from build123d import *

# Parameters (mm, degrees)
BOSS_EXTRUDE1_DEPTH = 12.446
SKETCH2_R           = 1.450000021
SKETCH2_R_2         = 2.900000042
CUT_EXTRUDE1_DEPTH  = 100.851652202
CHAMFER2_SIZE       = 0.5
CHAMFER3_SIZE       = 1


with BuildPart() as part:
    # Sketch1 → Boss-Extrude1 (new body)
    with BuildSketch(Plane.XY):
        Polygon((0, 8.001), (-41.850200018, 8.001), (-41.850200018, 16.256), (-57.090200018, 16.256), (-82.490200018, 16.256), (-97.730200018, 16.256), (-97.730200018, 8.001), (-97.730200018, -4.699), (-82.490200018, -4.699), (-82.490200018, 8.001), (-54.550200018, 8.001), (-54.550200018, -4.699), (-39.310200018, -4.699), (-39.310200018, 3.302), (-7.874, 3.302), (-7.874, 0), (0, 0), align=None)
    extrude(amount=BOSS_EXTRUDE1_DEPTH)

    # Sketch2 → Cut-Extrude1 (cut, through all)
    with BuildSketch(Plane.XZ):
        with Locations(Location((-90.110200018, 6.223, 0), (0, 0, 270))):
            Circle(SKETCH2_R)
        with Locations(Location((-46.930200018, 6.223, 0), (0, 0, 270))):
            Circle(SKETCH2_R_2)
        with Locations(Location((-3.937, 6.223, 0), (0, 0, 270))):
            Circle(SKETCH2_R)
    extrude(amount=-CUT_EXTRUDE1_DEPTH, mode=Mode.SUBTRACT)

    # Chamfer2
    chamfer2_edges = [part.edges().sort_by_distance(p)[0] for p in [
        (-90.110200018, 16.256, 7.673000021),
        (-3.937, 8.001, 7.673000021),
    ]]
    chamfer(chamfer2_edges, length=CHAMFER2_SIZE)

    # Chamfer3
    chamfer3_edges = [part.edges().sort_by_distance(p)[0] for p in [
        (-46.930200018, 16.256, 9.123000042),
    ]]
    chamfer(chamfer3_edges, length=CHAMFER3_SIZE)


solid = part.part
Work out the finished part from the listing and answer in its coordinate system (mm). A direction names the side the tool comes from. Coordinates: 2 decimals unless noted, no trailing zeros. Order: outer loops, then holes, each group sorted by start corner. A loop starts at its lowest first (then second) coordinate and runs counter-clockwise, first axis right, second up. Notation, with made-up numbers: (8, 3.5) - (51, 3.5) arc R22 cw to (51, 32.5) - close; hole circle Ø2 at (77.5, 87). An arc over 180 degrees is marked (long way). Put each result on its own line as item: value. Start each with the question number.
1) Find section C-C (z = 11). Give the vertices of the cut face in (x, y).
2) Find the intervals of material crossed by line 1 (X direction, y = 7.75, z = 2.25); line 2 (X direction, y = -0.75, z = 0.75); line 3 (X direction, y = 3.75, z = 6), in increasing order. Write a range as from..to.
3) Find section B-B (y = 6). Give the vertices of the cut face in (x, z), plus the area to 3 significant figures.
4) Flat-ended cylindrical pins translate along their axes: pin 1 (3.5 mm diameter, centred on x = -65.5, z = 9, fed in from -Y); pin 2 (0.9 mm diameter, centred on x = -91, z = 7, fed in from +Y); pin 3 (4 mm diameter, centred on x = -5, z = 8, fed in from -Y). Find the tip coordinate at first contact, or state that the pin passes through.
5) For a pull along Z with two mould halves and no side action, classify faces 1 (the flat face through (-60.4, 8.3, 0)), 2 (the flat face through (-90, -4.699, 6)), 3 (the flat face through (-47, 0, 6)) as released by +Z, released by -Z, zero draft, split by the parting line, or undercut.
6) Find section A-A (y = -2.25). Give the vertices of the cut face in (x, z).
7) For faces 4 (the flat face through (-24, 3.302, 6)), 5 (the flat face through (-47, -4.699, 6)), 6 (the flat face through (-21, 8.001, 6)), 7 (the flat face through (-90, 0, 6)), determine the directions among +Z, -Z, +X, -X, +Y, -Y from which every point of the face is accessible in a straight line to the end or side of a thin tool.
8) Find section D-D (x = -62.5). Give the vertices of the cut face in (y, z), plus the area to 3 significant figures.
Results list:
1. outline: (-97.73, -4.7) - (-82.49, -4.7) - (-82.49, 8) - (-54.55, 8) - (-54.55, -4.7) - (-39.31, -4.7) - (-39.31, 3.3) - (-7.87, 3.3) - (-7.87, 0) - (0, 0) - (0, 8) - (-41.85, 8) - (-41.85, 16.26) - (-97.73, 16.26) - close
2. line 1: x = -97.73..-82.49, -54.55..0
2. line 2: x = -97.73..-82.49, -54.55..-39.31
2. line 3: x = -97.73..-91.54, -88.68..-82.49, -54.55..-49.82, -44.04..-5.37, -2.5..0
3. outline: (-97.73, 0) - (-82.49, 0) - (-82.49, 12.45) - (-97.73, 12.45) - close; (-54.55, 0) - (0, 0) - (0, 12.45) - (-54.55, 12.45) - close; hole circle Ø2.9 at (-90.11, 6.22); hole circle Ø5.8 at (-46.93, 6.22); hole circle Ø2.9 at (-3.94, 6.22)
3. area: 829 mm^2
4. pin 1: stops at y = 8
4. pin 2: stops at y = 15.94
4. pin 3: stops at y = 0
5. face 1: released by -Z
5. face 2: zero draft
5. face 3: undercut
6. outline: (-97.73, 0) - (-82.49, 0) - (-82.49, 12.45) - (-97.73, 12.45) - close; (-54.55, 0) - (-39.31, 0) - (-39.31, 12.45) - (-54.55, 12.45) - close
7. face 4: +Z, -Z, -Y
7. face 5: +Z, -Z, +X, -X, -Y
7. face 6: +Z, -Z, +X, +Y
7. face 7: +Y
8. outline: (8, 0) - (16.26, 0) - (16.26, 12.45) - (8, 12.45) - close
8. area: 103 mm^2
